Part model, mm, in its own coordinate system. Face numbers are marked on the shaded views. A direction names the side the tool comes from. Give positions to 0.01 mm unless a question says otherwise; leave off trailing zeros. Order: outer loops, then holes, each group sorted by start corner. A loop starts at its lowest first (then second) coordinate and runs counter-clockwise, first axis right, second up. Notation, with made-up numbers: (18.25, 50) - (51.25, 50) arc R26 cw to (51.25, 64) - close; hole circle Ø3 at (75.25, 82). An arc over 180 degrees is marked (long way). One line per item, written item: value.
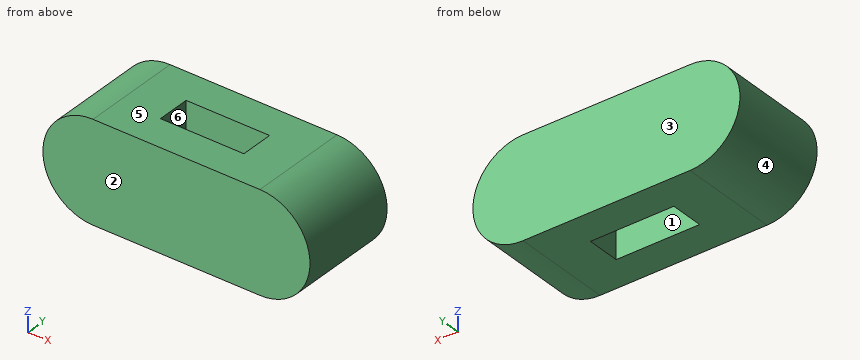
```python
from build123d import *

# Parameters (mm, degrees)
BOX001_W          = 5
BOX001_H          = 2
BOX001_DEPTH      = 6
CYLINDER001_R     = 3
CYLINDER001_DEPTH = 6
BOX_W             = 10
BOX_H             = 6
BOX_DEPTH         = 6
CYLINDER_R        = 3
CYLINDER_DEPTH    = 6


with BuildPart() as insert:
    # Box001 → Box001 (new body)
    with BuildSketch(Plane(origin=(-2.5, -1, 0), x_dir=(1, 0, 0), z_dir=(0, 0, 1))):
        with Locations((2.5, 1)):
            Rectangle(BOX001_W, BOX001_H)
    extrude(amount=BOX001_DEPTH)


with BuildPart() as obj1:
    # Cylinder001 → Cylinder001 (new body)
    with BuildSketch(Plane(origin=(5, 3, 0), x_dir=(1, 0, 0), z_dir=(0, -1, 0))):
        Circle(CYLINDER001_R)
    extrude(amount=CYLINDER001_DEPTH)


with BuildPart() as obj2:
    # Box → Box (new body)
    with BuildSketch(Plane(origin=(-5, -3, -3), x_dir=(1, 0, 0), z_dir=(0, 0, 1))):
        with Locations((5, 3)):
            Rectangle(BOX_W, BOX_H)
    extrude(amount=BOX_DEPTH)


with BuildPart() as obj3:
    # Cylinder → Cylinder (new body)
    with BuildSketch(Plane(origin=(-5, 3, 0), x_dir=(1, 0, 0), z_dir=(0, -1, 0))):
        Circle(CYLINDER_R)
    extrude(amount=CYLINDER_DEPTH)

    # Fusion: union obj1, obj2
    add(obj1.part)
    add(obj2.part)


with BuildPart() as obj3_1:
    # Fusion placement: moved
    add(obj3.part.moved(Location((0, 0, 3))))

    # Cut: cut Insert
    add(insert.part, mode=Mode.SUBTRACT)


solid = obj3_1.part
```
1) Which spindle directions (+Z, -Z, +X, -X, +Y, -Y) get a long thin tool onto all of the face, cutting with end or side? Do the marked faces 5 and 6. Say none if no direction does.
Answer:
face 5: +Z, +X, -X, +Y, -Y
face 6: +Z, -Z
2) Slice it at B-B on y = -0.25. Write the cut outline in (x, z), then the cut area to 3 significant figures.
Answer:
outline: (-5, 0) - (-2.5, 0) - (-2.5, 6) - (-5, 6) arc R3 ccw to start; (2.5, 0) - (5, 0) arc R3 ccw to (5, 6) - (2.5, 6) - close
area: 58.3 mm2
3) Slice it at C-C on z = 4. Write the cut outline in (x, y).
Answer:
outline: (-7.83, -3) - (7.83, -3) - (7.83, 3) - (-7.83, 3) - close; hole (-2.5, -1) - (2.5, -1) - (2.5, 1) - (-2.5, 1) - close
4) Two-plate mould, pull along Y, no slides. Class the marked faces 1, 2, 3 and 4: pulls with the +Y half, pulls with the -Y half, needs draft (parallel to the pull), parting line crosses it, or undercut.
Answer:
face 1: undercut
face 2: pulls with the -Y half
face 3: pulls with the +Y half
face 4: needs draft
5) Wall check: line 1 along Y through (x, z) = (-2, 1.8); line 2 along X through (y, z) = (-0.3, 4.2); line 3 along X through (y, z) = (-0.7, 0.4). Give the ranges that are in metal, low to high. Write a range as [from, to].
Answer:
line 1: y = [-3, -1], [1, 3]
line 2: x = [-7.75, -2.5], [2.5, 7.75]
line 3: x = [-6.5, -2.5], [2.5, 6.5]
6) Drop flat-ended pins along their axis: P1, Ø1, axis at y = 0, z = 2.5, coming from the +X side; P2, Ø1, axis at y = 0, z = 4, coming from the -X side. Give the stop position or say it passes through.
Answer:
P1: stops at x = 8
P2: stops at x = -7.96
7) Slice it at A-A on x = -2. Write the cut outline in (y, z).
Answer:
outline: (-3, 0) - (-1, 0) - (-1, 6) - (-3, 6) - close; (1, 0) - (3, 0) - (3, 6) - (1, 6) - close
